Autodesk Inventor part; units mm, degrees
ref_plane "YZ Plane" through (0, 0, 0) normal (1, 0, 0) x (0, 1, 0)
ref_plane "XZ Plane" through (0, 0, 0) normal (0, 1, 0) x (-1, 0, 0)
ref_plane "XY Plane" through (0, 0, 0) normal (0, 0, 1) x (1, 0, 0)
sketch "Sketch2" plane through (0, 0, 0) normal (0, 1, 0) x (-1, 0, 0)
  line L0 (0, 0) -> (-36, 0)
  line L1 (-36, 0) -> (-36, -100)
  line L2 (-36, -100) -> (0, -100)
  line L3 (0, -100) -> (0, 0)
  line L4 (-36, 0) -> (-36, -20)
  line L5 (-36, -20) -> (0, -20)
  line L6 (-36, -100) -> (-36, -80)
  line L7 (-36, -80) -> (-36, -61.7109)
  line L8 (0, -61.7109) -> (0, -80)
  line L9 (-36, -80) -> (-36, -70)
  line L10 (-36, -70) -> (0, -70)
  line L11 (0, -80) -> (-36, -80)
  line L12 (0, -70) -> (0, -80)
  line L13 (0, -70) -> (-5, -70)
  line L14 (-5, -70) -> (-5, -80)
  line L15 (-36, -20) -> (-36, -30)
  line L16 (-36, -30) -> (0, -30)
  line L17 (0, -20) -> (-5, -20)
  line L18 (-5, -20) -> (-5, -30)
  line L19 (-36, -80) -> (-31, -80)
  line L20 (-31, -80) -> (-31, -70)
  line L21 (-31, -30) -> (-31, -20)
  line L22 (-18, 0) -> (-18, -15)
  circle A0 centre (-18, -15) radius 12
  line L23 (-18, -15) -> (-18, -45.5)
  line L24 (-18, -45.5) -> (-18, -86)
  line L25 (-18, -15) -> (-18, -45)
  circle A1 centre (-18, -45) radius 5.05
  line L26 (-18, -45) -> (-18, -85)
  circle A2 centre (-18, -85) radius 5.05
  dimension "d0" = 36
  dimension "d1" = 100
  dimension "d2" = 20
  dimension "d3" = 20
  dimension "d4" = 10
  dimension "d5" = 5
  dimension "d6" = 10
  dimension "d7" = 5
  dimension "d8" = 5
  dimension "d9" = 15
  dimension "d10" = 24
  dimension "d17" = 30
  dimension "d18" = 10.1
  dimension "d19" = 40
  dimension "d20" = 10.1
extrude "Extrusion1" add sketch "Sketch2" along normal blind 5 contours L3 L5 A0 L22 L0 | L22 A0 L5 L1 L0 | L3 L10 L24 A1 L23 L16 | L18 L16 L23 A0 L5 | A0 L23 L16 L21 L5 | L16 L23 A1 L24 L10 L1 | L3 L2 L1 L11 A2 | L14 L11 A2 L24 L10 | L24 A2 L11 L20 L10
sketch "Sketch3" plane through (0, 5, 0) normal (0, 1, 0) x (1, 0, 0)
  circle A0 centre (18, 45) radius 5.05
  circle A1 centre (18, 45) radius 5.05
  circle A2 centre (18, 45) radius 2.25
  circle A3 centre (18, 85) radius 5.05
  circle A4 centre (18, 85) radius 5.05
  circle A5 centre (18, 85) radius 2.25
  point P0 (0, 0)
  dimension "d21" = 4.5
  dimension "d22" = 4.5
extrude "Extrusion2" add sketch "Sketch3" against normal blind 1
equation "\"BendRadius\" = Thickness"
equation "\"BendReliefWidth\" = Thickness"
equation "\"BendReliefDepth\" = 0.5 * Thickness"
equation "\"CornerReliefSize\" = 4 * Thickness"
equation "\"MinimumRemnant\" = 2 * Thickness"
equation "\"TransitionRadius\" = BendRadius"
equation "\"JacobiRadiusSize\" = BendRadius"
equation "\"GapSize\" = Thickness"
properties part number "Part2v2"
Read the model definition and answer for the solid it produces. Units are mm, in the model's axes. A direction names the side the tool comes from. Coordinates: 2 decimals unless noted, no trailing zeros. Write each loop counter-clockwise with the first axis right and the second up, starting at its lowest first coordinate (ties: lowest second). Pieces come first, ordered by that corner, then holes. Notation, with made-up numbers: (12, 17.5) -> (54, 17.5) arc R8 ccw to (54, 25.5) -> close; hole circle Ø1 at (-35, 88). An arc over 180 degrees is marked (long way). Write item = value, one per line.
(1) Straight lines are drawn through the part: L1, parallel to Z at x = 18, y = 1.1; L2, parallel to Z at x = 18, y = 4.4; L3, parallel to Z at x = 2.5, y = 3.25. For each, find the intervals that lie inside material, in ascending order. Write a range as from..to.
From the geometry:
L1 = -100..-90.05, -79.95..-50.05, -39.95..-27, -3..0
L2 = -100..-87.25, -82.75..-47.25, -42.75..-27, -3..0
L3 = -100..-80, -70..-30, -20..0
(2) Section B-B on x = 18 is taken. Write down the section's boundary in (y, z), plus the area to 3 significant figures.
From the geometry:
outline = (0, -100) -> (5, -100) -> (5, -87.25) -> (4, -87.25) -> (4, -90.05) -> (0, -90.05) -> close; (0, -79.95) -> (4, -79.95) -> (4, -82.75) -> (5, -82.75) -> (5, -47.25) -> (4, -47.25) -> (4, -50.05) -> (0, -50.05) -> close; (0, -39.95) -> (4, -39.95) -> (4, -42.75) -> (5, -42.75) -> (5, -27) -> (0, -27) -> close; (0, -3) -> (5, -3) -> (5, 0) -> (0, 0) -> close
area = 290 mm2
(3) Section C-C on y = 1.15 is taken. Write down the section's boundary in (x, z).
From the geometry:
outline = (0, -100) -> (36, -100) -> (36, -80) -> (31, -80) -> (31, -70) -> (36, -70) -> (36, -30) -> (31, -30) -> (31, -20) -> (36, -20) -> (36, 0) -> (0, 0) -> (0, -20) -> (5, -20) -> (5, -30) -> (0, -30) -> (0, -70) -> (5, -70) -> (5, -80) -> (0, -80) -> close; hole circle Ø24 at (18, -15); hole circle Ø10.1 at (18, -85); hole circle Ø10.1 at (18, -45)
(4) Which of the six approach directions +Z, -Z, +X, -X, +Y, -Y give full straight-line access (tool end or side, diameter ignored) to faces 4 (the face through (34, 2, -20)), 5 (the face through (3, 2, -30)), 6 (the face through (22, 0, -49)), 7 (the face through (18, 2, -100)), 8 (the face through (22.01, 1.97, -41.93))?
From the geometry:
face_4 = +X, +Y, -Y
face_5 = -X, +Y, -Y
face_6 = +Z, -Z, +X, -X, -Y
face_7 = -Z, +X, -X, +Y, -Y
face_8 = -Y
(5) For a pull along X with two mould halves and no side action, classify faces 1 (the face through (2, 2, -80)), 2 (the face through (5, 2, -25)), 3 (the face through (19.21, 4.507, -46.897)) as +X half, -X half, draft (parallel to the pull), parting line (faces both ways), or undercut.
From the geometry:
face_1 = draft
face_2 = -X half
face_3 = undercut
(6) Section A-A on z = -85 is taken. Write down the section's boundary in (x, y).
From the geometry:
outline = (0, 0) -> (12.95, 0) -> (12.95, 4) -> (15.75, 4) -> (15.75, 5) -> (0, 5) -> close; (20.25, 4) -> (23.05, 4) -> (23.05, 0) -> (36, 0) -> (36, 5) -> (20.25, 5) -> close
(7) Given pin 1 Ø2.5 at (y, z) = (3.5, -23) entering from -X; pin 2 Ø3.5 at (x, z) = (18, -45) entering from -Y; pin 3 Ø8 at (x, z) = (18, -85) entering from -Y; pin 4 Ø1.5 at (y, z) = (2.5, -25) entering from +X, each flat-ended and moving along its own axis, determine where each tip first touches the part or whether it passes through.
From the geometry:
pin_1 = 5
pin_2 = through
pin_3 = 4
pin_4 = 31
(8) Section D-D on z = -16 is taken. Write down the section's boundary in (x, y), plus the area to 3 significant figures.
From the geometry:
outline = (0, 0) -> (6.04, 0) -> (6.04, 5) -> (0, 5) -> close; (29.96, 0) -> (36, 0) -> (36, 5) -> (29.96, 5) -> close
area = 60.4 mm2
